```python
from build123d import *

# Parameters (mm, degrees)
F1_DEPTH = 25
F3_W     = 3.1
F3_H     = 395.207942
F4_DEPTH = 153
F5_R     = 10


with BuildPart() as f1:
    # F0 (on Front) → F1 (new body)
    with BuildSketch(Plane.XZ):
        Polygon((0, 0), (93.106838, 0), (105.260208, 0), (98.35337, 10), (0, 152.4), align=None)
        Polygon((10, 10), (10, 120.325452), (86.2, 10), align=None, mode=Mode.SUBTRACT)
    extrude(amount=F1_DEPTH)

    # F3 (on offset) → F4 (cut, through all)
    with BuildSketch(Plane.YZ.offset(163)):
        with Locations((-12.5, 0)):
            Rectangle(F3_W, F3_H)
    extrude(amount=-F4_DEPTH, mode=Mode.SUBTRACT)

    # F5
    f5_edges = [f1.edges().sort_by_distance(p)[0] for p in [
        (105.260208, -19.525, 0),
        (105.260208, -5.475, 0),
        (10, -19.525, 10),
        (10, -5.475, 10),
        (10, -19.525, 120.325452),
        (10, -5.475, 120.325452),
        (86.2, -19.525, 10),
        (86.2, -5.475, 10),
    ]]
    fillet(f5_edges, radius=F5_R)


solid = f1.part
```
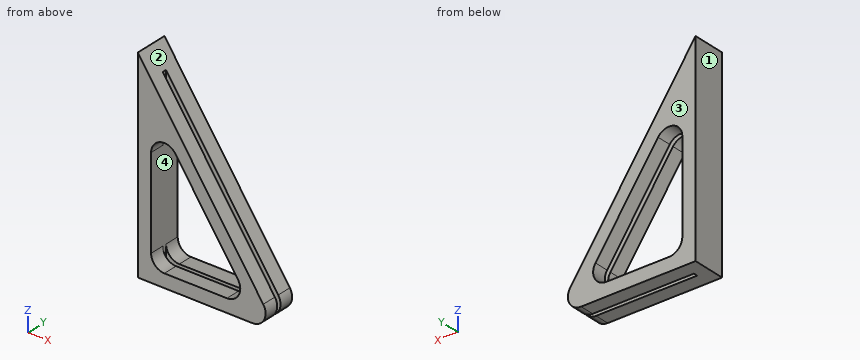
The model under review builds one solid part; all positions refer to its coordinate system, in mm. Face numbers are marked on the shaded views. Round coordinates to 2 decimals unless told otherwise and drop trailing zeros. Order: outer loops, then holes, each group sorted by start corner. A loop starts at its lowest first (then second) coordinate and runs counter-clockwise, first axis right, second up.
(1) Take a section at A-A, the plane z = 55. State the section outline as (x, y) points.
Working result:
outline: (0, -25) - (10, -25) - (10, 0) - (0, 0) - close; (55.12, -25) - (67.27, -25) - (67.27, -14.05) - (55.12, -14.05) - close; (55.12, -10.95) - (67.27, -10.95) - (67.27, 0) - (55.12, 0) - close
(2) Mouldability with a two-part tool opening along X and no side actions: class the marked faces 1, 2, 3 and 4 as released by +X, released by -X, zero draft, split by the parting line, or undercut.
Working result:
face 1: released by -X
face 2: released by +X
face 3: zero draft
face 4: undercut
(3) Wall thickness on L1, parallel to Y at x = 81, z = 33.5; L2, parallel to Z at x = 59.5, y = -15.25: over which ranges is each line inside the solid? List them lowest first.
Working result:
L1: y = -25 to -14.05, -10.95 to 0
L2: z = 0 to 10, 48.66 to 66.25
(4) Take a section at C-C, the plane x = 84. State the section outline as (y, z) points, plus the area to 3 significant figures.
Working result:
outline: (-25, 0) - (-14.05, 0) - (-14.05, 30.78) - (-25, 30.78) - close; (-10.95, 0) - (0, 0) - (0, 30.78) - (-10.95, 30.78) - close
area: 674 mm2
(5) Take a section at B-B, the plane x = 69. State the section outline as (y, z) points, plus the area to 3 significant figures.
Working result:
outline: (-25, 0) - (-14.05, 0) - (-14.05, 10.17) - (-25, 10.17) - close; (-25, 34.9) - (-14.05, 34.9) - (-14.05, 52.5) - (-25, 52.5) - close; (-10.95, 0) - (0, 0) - (0, 10.17) - (-10.95, 10.17) - close; (-10.95, 34.9) - (0, 34.9) - (0, 52.5) - (-10.95, 52.5) - close
area: 608 mm2
(6) Take a section at D-D, the plane z = 130. State the section outline as (x, y) points.
Working result:
outline: (0, -25) - (15.47, -25) - (15.47, -14.05) - (10, -14.05) - (10, -10.95) - (15.47, -10.95) - (15.47, 0) - (0, 0) - close
(7) For P1, Ø12, axis at y = -3.5, z = 101, coming from the +X side; P2, Ø2, axis at y = -9.5, z = 88.5, coming from the +X side; P3, Ø9, axis at x = 37.5, y = -17, coming from the +Z side, all flat-tipped, find the tip position at first contact; note any pin that passes through.
Working result:
P1: stops at x = 39.65
P2: stops at x = 44.83
P3: stops at z = 104.62
